Autodesk Inventor part; units mm, degrees
ref_plane "YZ Plane" through (0, 0, 0) normal (1, 0, 0) x (0, 1, 0)
ref_plane "XZ Plane" through (0, 0, 0) normal (0, 1, 0) x (-1, 0, 0)
ref_plane "XY Plane" through (0, 0, 0) normal (0, 0, 1) x (1, 0, 0)
sketch "Sketch1" plane through (0, 0, 0) normal (0, 1, 0) x (-1, 0, 0)
  line L0 (75, 75) -> (-75, 75)
  line L1 (-75, 75) -> (-75, -75)
  line L2 (-75, -75) -> (75, -75)
  line L3 (75, -75) -> (75, 75)
  line L4 (75, 75) -> (-75, -75) construction
  line L5 (-75, 75) -> (75, -75) construction
  point P0 (0, 0)
  dimension "d0" = 150
  dimension "d1" = 150
extrude "Extrusion1" add sketch "Sketch1" along normal blind 5
sketch "Sketch2" plane through (0, 5, 0) normal (0, 1, 0) x (1, 0, 0)
  line L0 (10, -55) -> (-10, -55)
  line L1 (-10, -55) -> (-10, -35)
  line L2 (-10, -35) -> (10, -35)
  line L3 (10, -35) -> (10, -55)
  line L4 (10, -55) -> (-10, -35) construction
  line L5 (-10, -55) -> (10, -35) construction
  line L6 (-75, -75) -> (75, -75)
  point P0 (0, 0)
  point P1 (0, -45)
  dimension "d4" = 20
  dimension "d5" = 20
  dimension "d6" = 20
extrude "Extrusion2" add sketch "Sketch2" along normal blind 10
fillet "Fillet1" radius 5 12 edges at (75, 2.5, 75) (75, 2.5, -75) (-75, 2.5, 75) (-75, 2.5, -75) (10, 10, 55) (10, 10, 35) (-10, 10, 35) (-10, 10, 55) (-10, 15, 45) (0, 15, 55) (10, 15, 45) (0, 15, 35)
fillet "Fillet2" radius 2 16 edges at (73.5355, 5, -73.5355) (0, 5, -75) (-73.5355, 5, -73.5355) (-75, 5, 0) (-73.5355, 5, 73.5355) (0, 5, 75) (73.5355, 5, 73.5355) (75, 5, 0) (73.5355, 0, -73.5355) (0, 0, -75) (-73.5355, 0, -73.5355) (-75, 0, 0) (-73.5355, 0, 73.5355) (0, 0, 75) (73.5355, 0, 73.5355) (75, 0, 0)
properties part number "slider"
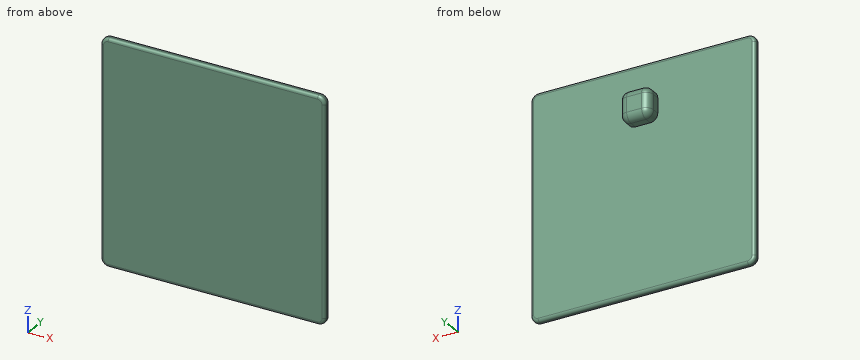
The model under review builds one solid part; all positions refer to its coordinate system, in mm. Give positions to 0.01 mm unless a question says otherwise; leave off trailing zeros. Write each loop counter-clockwise with the first axis right and the second up, starting at its lowest first coordinate (ties: lowest second). Pieces come first, ordered by that corner, then holes.
1. Add section A-A, the plane z = 53. Write out the cut boundary in (x, y), plus the area to 3 significant figures.
2. For P1, Ø3, axis at x = -48, z = -39.5, coming from the +Y side; P2, Ø5, axis at y = 5, z = 37.5, coming from the +X side; P3, Ø4, axis at y = 6.5, z = 44.5, coming from the +X side; P4, Ø2.5, axis at y = 6.5, z = 46.5, coming from the -X side, all flat-tipped, find the tip position at first contact; note any pin that passes through.
3. Add section B-B, the plane y = 6.75. Write out the cut boundary in (x, z).
4. Wall thickness on L1, parallel to Y at x = -68, z = -66; L2, parallel to X at y = 12, z = 54; L3, parallel to Z at x = 3, y = 4.75: over which ranges is each line inside the solid? List them lowest first.
5. Add section C-C, the plane x = 49.5. Write out the cut boundary in (y, z), plus the area to 3 significant figures.
Worked answers:
1. outline: (-75, 2) arc R2 ccw to (-73, 0) - (73, 0) arc R2 ccw to (75, 2) - (75, 3) arc R2 ccw to (73, 5) - (9, 5) - (9, 10) arc R4 ccw to (5, 14) - (-5, 14) arc R4 ccw to (-9, 10) - (-9, 5) - (-73, 5) arc R2 ccw to (-75, 3) - close
1. area: 902 mm2
2. P1: stops at y = 5
2. P2: stops at x = 75
2. P3: stops at x = 74.32
2. P4: stops at x = -10
3. outline: (-10, 40) arc R5 ccw to (-5, 35) - (5, 35) arc R5 ccw to (10, 40) - (10, 50) arc R5 ccw to (5, 55) - (-5, 55) arc R5 ccw to (-10, 50) - close
4. L1: y = 0 to 5
4. L2: x = -7.24 to 7.24
4. L3: z = -73.97 to 73.97
5. outline: (0, -73) arc R2 ccw to (2, -75) - (3, -75) arc R2 ccw to (5, -73) - (5, 73) arc R2 ccw to (3, 75) - (2, 75) arc R2 ccw to (0, 73) - close
5. area: 747 mm2
